from build123d import *

# Parameters (mm, degrees)
F1_DEPTH = 25.4


with BuildPart() as f1:
    # F0 (on Top) → F1 (new body)
    with BuildSketch(Plane.XY):
        with BuildLine():
            ThreePointArc((35.357989, -55.773497), (34.700263, -57.288462), (33.846916, -58.702506))
            ThreePointArc((33.846916, -58.702506), (30.076924, -64.689377), (24.690598, -69.276638))
            ThreePointArc((24.690598, -69.276638), (18.00206, -75.151493), (11.039559, -80.69893))
            ThreePointArc((11.039559, -80.69893), (10.464903, -83.658978), (11.039559, -86.619027))
            ThreePointArc((11.039559, -86.619027), (13.021343, -85.560107), (14.03443, -83.554506))
            ThreePointArc((14.03443, -83.554506), (20.760438, -77.35253), (29.357025, -74.221656))
            ThreePointArc((29.357025, -74.221656), (40.186668, -71.149018), (49.206674, -64.413905))
            ThreePointArc((49.206674, -64.413905), (67.765139, -66.686066), (86.39013, -65.046228))
            ThreePointArc((86.39013, -65.046228), (90.842719, -66.681712), (94.834223, -69.244571))
            ThreePointArc((94.834223, -69.244571), (93.58406, -71.906754), (91.913037, -74.327044))
            ThreePointArc((91.913037, -74.327044), (89.952947, -73.623328), (87.874644, -73.489815))
            ThreePointArc((87.874644, -73.489815), (85.993248, -75.819788), (85.806198, -78.808673))
            ThreePointArc((85.806198, -78.808673), (90.243806, -78.661543), (94.375476, -77.035718))
            ThreePointArc((94.375476, -77.035718), (94.732683, -77.994564), (95.723428, -78.250311))
            ThreePointArc((95.723428, -78.250311), (99.839405, -77.015924), (103.444606, -74.677654))
            ThreePointArc((103.444606, -74.677654), (105.422994, -70.957733), (106.698684, -66.942208))
            ThreePointArc((106.698684, -66.942208), (106.805126, -64.950848), (106.006868, -63.123383))
            ThreePointArc((106.006868, -63.123383), (100.195754, -61.321046), (94.247706, -60.04113))
            ThreePointArc((94.247706, -60.04113), (95.936674, -54.912618), (95.482543, -49.532283))
            ThreePointArc((95.482543, -49.532283), (98.447384, -44.774679), (101.387411, -40.001702))
            ThreePointArc((101.387411, -40.001702), (105.597536, -41.38767), (109.645344, -43.193579))
            ThreePointArc((109.645344, -43.193579), (111.519486, -43.779772), (113.393627, -43.193579))
            ThreePointArc((113.393627, -43.193579), (117.01848, -41.827539), (115.970574, -38.098261))
            ThreePointArc((115.970574, -38.098261), (113.180417, -35.898183), (110.64098, -33.412911))
            ThreePointArc((110.64098, -33.412911), (108.327022, -29.635914), (104.550026, -27.321953))
            ThreePointArc((104.550026, -27.321953), (106.217319, -24.648898), (109.025061, -23.220027))
            ThreePointArc((109.025061, -23.220027), (111.496496, -20.781246), (112.031601, -17.350603))
            ThreePointArc((112.031601, -17.350603), (110.113696, -16.106507), (109.025061, -18.116733))
            ThreePointArc((109.025061, -18.116733), (107.794978, -20.560822), (105.402686, -21.888833))
            ThreePointArc((105.402686, -21.888833), (101.226365, -22.791684), (97.81839, -20.214379))
            ThreePointArc((97.81839, -20.214379), (97.040255, -16.635745), (99.689841, -14.107542))
            ThreePointArc((99.689841, -14.107542), (103.139321, -13.121868), (104.59435, -9.842637))
            ThreePointArc((104.59435, -9.842637), (102.452988, -8.646448), (100.360706, -9.926547))
            ThreePointArc((100.360706, -9.926547), (99.206159, -10.920505), (97.81839, -11.549016))
            ThreePointArc((97.81839, -11.549016), (97.7106, -10.42277), (98.19214, -9.39897))
            ThreePointArc((98.19214, -9.39897), (97.297537, -7.296311), (95.162444, -8.110479))
            ThreePointArc((95.162444, -8.110479), (94.347536, -9.733247), (94.326667, -11.549016))
            ThreePointArc((94.326667, -11.549016), (91.24145, -11.077832), (88.122092, -10.976911))
            ThreePointArc((88.122092, -10.976911), (87.140114, -11.893801), (87.481856, -13.193102))
            ThreePointArc((87.481856, -13.193102), (90.208654, -14.483161), (93.213789, -14.745539))
            ThreePointArc((93.213789, -14.745539), (92.91737, -20.129205), (95.723428, -24.733309))
            ThreePointArc((95.723428, -24.733309), (94.196841, -26.440721), (91.913037, -26.613809))
            ThreePointArc((91.913037, -26.613809), (89.720804, -27.125156), (89.744188, -29.376114))
            ThreePointArc((89.744188, -29.376114), (93.548656, -30.795), (97.353123, -29.376114))
            ThreePointArc((97.353123, -29.376114), (97.623646, -29.667451), (97.814836, -30.016029))
            ThreePointArc((97.814836, -30.016029), (92.320304, -34.797902), (87.223575, -40.001702))
            ThreePointArc((87.223575, -40.001702), (74.926958, -45.213773), (61.732344, -47.281299))
            ThreePointArc((61.732344, -47.281299), (49.657937, -45.265171), (37.58353, -47.281299))
            ThreePointArc((37.58353, -47.281299), (31.965668, -48.141093), (27.217193, -51.263846))
            ThreePointArc((27.217193, -51.263846), (26.912313, -54.662213), (30.26267, -54.01649))
            ThreePointArc((30.26267, -54.01649), (33.073036, -51.058678), (37.114996, -50.502479))
            ThreePointArc((37.114996, -50.502479), (36.047411, -53.074961), (35.357989, -55.773497))
        make_face()
    extrude(amount=F1_DEPTH)


solid = f1.part
CAD build for the part. Positions are in the model's coordinates, mm. A direction names the side the tool comes from. Give positions to 0.01 mm unless a question says otherwise; leave off trailing zeros. Write each loop counter-clockwise with the first axis right and the second up, starting at its lowest first coordinate (ties: lowest second). Pieces come first, ordered by that corner, then holes. Notation, with made-up numbers: M 52.5,1 L 71.5,1 A4 cw 71.5,5 Z; hole C -36.5,6.5 d11. An arc over 180 degrees is marked long. Put each result on its own line as item: value. Start each with the question number.
(1) Which spindle directions (+Z, -Z, +X, -X, +Y, -Y) get a long thin tool onto all of the face, cutting with end or side? Do faces 4 (the face through (102.489, -8.646, 12.522)), 5 (the face through (40.04, -71.22, 12.52)), 6 (the face through (101.287, -22.805, 12.522)), 7 (the face through (76, -53, 0)), 8 (the face through (108.37, -29.68, 12.52)). Say none if no direction does.
(2) Probe L1, parallel to Y at x = 87.5, z = 3.25; L2, parallel to Y at x = 96.5, z = 11.5; L3, parallel to X at y = -49.5, z = 23.5. List the from-to ranges inside material, lowest first.
(3) Band-saw the part on B-B, the plane y = -57.5. Write the cut outline in (x, z), and give its area (3 significant figures).
(4) Flat gauge pins, fed straight in: pin 1 Ø12 at (x, z) = (70.5, 10) entering from +Y; pin 2 Ø12 at (x, z) = (78.5, 9.5) entering from +Y; pin 3 Ø12 at (x, z) = (23.5, 15.5) entering from -Y. Where does each tip first touch, or does it go through?
(5) Mould opens along X. For faces 1 (the face through (105.4, -71.01, 12.52)), 2 (the face through (111.49, -43.78, 12.52)), 3 (the face through (30.142, -64.614, 12.522)) say: +X half, -X half, draft (parallel to the pull), parting line (faces both ways), or undercut.
(6) Band-saw the part on A-A, the plane x = 84. Write the cut outline in (y, z).
Response values:
1. face 4: +Z, -Z, +Y
1. face 5: +Z, -Z, -Y
1. face 6: +Z, -Z
1. face 7: -Z, +X, -X, +Y, -Y
1. face 8: +Z, -Z, +X
2. L1: y = -78.93 to -73.76, -65.35 to -39.7, -13.21 to -11.3
2. L2: y = -78.11 to -60.46, -47.91 to -31.09, -29.99 to -7.17
2. L3: x = 29.34 to 95.5
3. outline: M 34.59,0 L 95.37,0 L 95.37,25.4 L 34.59,25.4 Z
3. area: 1,540 mm2
4. pin 1: stops at y = -44.74
4. pin 2: stops at y = -41.47
4. pin 3: stops at y = -79.75
5. face 1: +X half
5. face 2: undercut
5. face 3: -X half
6. outline: M -65.48,0 L -41.72,0 L -41.72,25.4 L -65.48,25.4 Z
